The model under review builds one solid part; all positions refer to its coordinate system, in mm. A direction names the side the tool comes from. Give positions to 0.01 mm unless a question says otherwise; leave off trailing zeros. Loops run counter-clockwise (first coordinate to the right, second up) from the corner with the lowest first, then second, coordinate; pieces in that order, holes last. Notation, with made-up numbers: (-1.5, 10) - (12.5, 10) arc R8 ccw to (12.5, 21) - close; hole circle Ø8 at (-2.5, -20.75). An arc over 180 degrees is marked (long way). Return JSON: item names as keys, results as strings. Group by question number.
Autodesk Inventor part; units mm, degrees
ref_plane "YZ Plane" through (0, 0, 0) normal (1, 0, 0) x (0, 1, 0)
ref_plane "XZ Plane" through (0, 0, 0) normal (0, 1, 0) x (-1, 0, 0)
ref_plane "XY Plane" through (0, 0, 0) normal (0, 0, 1) x (1, 0, 0)
sketch "Sketch1" plane through (0, 0, 0) normal (0, 1, 0) x (-1, 0, 0)
  line L0 (0, 0) -> (25, 0)
  line L1 (25, 0) -> (25, -30)
  line L2 (25, -30) -> (0, -30)
  line L3 (0, -30) -> (0, 0)
  circle A0 centre (20, -4) radius 1.5
  circle A1 centre (20, -26) radius 1.5
  circle A2 centre (10, -4) radius 1.5
  circle A3 centre (10, -26) radius 1.5
  dimension "d0" = 30
  dimension "d1" = 25
  dimension "d2" = 3
  dimension "d5" = 22
  dimension "d8" = 10
  dimension "d11" = 20
  dimension "d12" = 4
extrude "Extrusion1" add sketch "Sketch1" along normal blind 25.5
sketch "Sketch2" plane through (0, 0, 0) normal (1, 0, 0) x (0, 0, -1)
  line L0 (0, 0) -> (30, 0)
  line L1 (30, 0) -> (30, 25.5)
  line L2 (0, 25.5) -> (30, 25.5)
  line L3 (0, 0) -> (0, 25.5)
  line L4 (8.25, 25.5) -> (21.75, 25.5)
  line L5 (21.75, 25.5) -> (21.75, 3)
  line L6 (21.75, 3) -> (8.25, 3)
  line L7 (8.25, 3) -> (8.25, 25.5)
  line L8 (30, 25.5) -> (0, 25.5)
  line L9 (30, 0) -> (30, 25.5)
  line L10 (24.15, 25.5) -> (30, 25.5)
  line L11 (30, 25.5) -> (30, 3)
  line L12 (30, 3) -> (24.15, 3)
  line L13 (24.15, 3) -> (24.15, 25.5)
  line L14 (0, 25.5) -> (5.85, 25.5)
  line L15 (5.85, 25.5) -> (5.85, 3)
  line L16 (5.85, 3) -> (0, 3)
  line L17 (0, 3) -> (0, 25.5)
  point P0 (0, 3)
  point P1 (30, 3)
  dimension "d15" = 3
  dimension "d16" = 3
  dimension "d17" = 3
  dimension "d19" = 13.5
  dimension "d20" = 2.4
  dimension "d21" = 2.4
  dimension "d22" = 5.85
extrude "Extrusion2" cut sketch "Sketch2" against normal blind 25.5 contours L3 L2 L15 L16 | L12 L13 L2 L1 | L2 L5 L6 L7
sketch "Sketch3" plane through (0, 3, -5.85) normal (0, 0, 1) x (1, 0, 0)
  circle A0 centre (-18, 8) radius 5
  line L0 (-25, 0) -> (-25, 22.5)
  line L1 (0, 0) -> (-25, 0)
  line L2 (0, 22.5) -> (0, 0)
  line L3 (-25, 22.5) -> (0, 22.5)
  line L4 (-25, 15) -> (-11, 15)
  line L5 (-11, 15) -> (0, 6)
  line L6 (0, 0) -> (0, 22.5)
  point P0 (0, -3)
  point P1 (0, 6)
  dimension "d25" = 8
  dimension "d26" = 7
  dimension "d27" = 7
  dimension "d28" = 14
  dimension "d29" = 6
  dimension "d30" = 10
extrude "Extrusion3" cut sketch "Sketch3" against normal blind 25.5 contours A0 | L0 L3 L2 L5 L4
fillet "Fillet1" radius 7 6 edges at (-25, 18, -22.95) (-11, 18, -22.95) (0, 9, -22.95) (-11, 18, -7.05) (0, 9, -7.05) (-25, 18, -7.05)
properties part number "beslag_board_3D"
Item 1: For L1, parallel to Z at x = -10, y = 1.25; L2, parallel to X at y = 1.05, z = -4; L3, parallel to Y at x = -18, z = -7.2, list the stretches that pass through material, from the lowest coordinate up. Write a range as from..to.
Item 2: Mouldability with a two-part tool opening along Y and no side actions: class faces 1 (the face through (-12, 9, -8.25)), 2 (the face through (-12, 3, -3)), 3 (the face through (-22, 14, -23)) as +Y half, -Y half, draft (parallel to the pull), parting line (faces both ways), or undercut.
Item 3: Take a section at C-C (z = -22.5). State the section outline as (x, y) points.
Item 4: Take a section at B-B (y = 13.5). State the section outline as (x, z) points.
Item 5: Take a section at A-A (z = -26). State the section outline as (x, y) points, then the cut area to 3 significant figures.
Item 6: Take a section at D-D (y = 1.75). State the section outline as (x, z) points, then the cut area to 3 significant figures.
Item 7: For P1, Ø3, axis at x = -21.5, y = 5.5, coming from the -Z side; P2, Ø3.5, axis at x = -10, z = -4, coming from the +Y side; P3, Ø5, axis at x = -10, z = -26, coming from the +Y side, all flat-tipped, find the tip position at first contact; note any pin that passes through.
Item 8: Tool access review of faces 4 (the face through (-12, 1, 0)), 5 (the face through (-12, 3, -27)), 6 (the face through (-11.177, 17.604, -7.067)), 7 (the face through (-12, 9, -5.85)), 8 (the face through (-12, 9, -21.75)): name each direction out of +Z, -Z, +X, -X, +Y, -Y from which nothing blocks a thin tool from reaching the whole face with its end or side.
Check sheet entries:
{
 "1": {"L1": "z = -30..-27.5, -24.5..-5.5, -2.5..0", "L2": "x = -25..-21.5, -18.5..-11.5, -8.5..0", "L3": "y = 0..6, 16..18"},
 "2": {"face 1": "draft", "face 2": "+Y half", "face 3": "undercut"},
 "3": {"outline": "(-25, 0) - (0, 0) - (0, 5.68) arc R7 ccw to (-2.57, 11.1) - (-9.07, 16.42) arc R7 ccw to (-13.5, 18) - (-18, 18) arc R7 ccw to (-25, 11) - close; hole circle Ø10 at (-18, 11)"},
 "4": {"outline": "(-24.54, -24.15) - (-22.33, -24.15) - (-22.33, -21.75) - (-24.54, -21.75) - close; (-24.54, -8.25) - (-22.33, -8.25) - (-22.33, -5.85) - (-24.54, -5.85) - close; (-13.67, -24.15) - (-5.5, -24.15) - (-5.5, -21.75) - (-13.67, -21.75) - close; (-13.67, -8.25) - (-5.5, -8.25) - (-5.5, -5.85) - (-13.67, -5.85) - close"},
 "5": {"outline": "(-25, 0) - (-21.5, 0) - (-21.5, 3) - (-25, 3) - close; (-18.5, 0) - (-11.5, 0) - (-11.5, 3) - (-18.5, 3) - close; (-8.5, 0) - (0, 0) - (0, 3) - (-8.5, 3) - close", "area": "57.0 mm^2"},
 "6": {"outline": "(-25, -30) - (0, -30) - (0, 0) - (-25, 0) - close; hole circle Ø3 at (-20, -26); hole circle Ø3 at (-20, -4); hole circle Ø3 at (-10, -26); hole circle Ø3 at (-10, -4)", "area": "722 mm^2"},
 "7": {"P1": "stops at z = -24.15", "P2": "stops at y = 3", "P3": "stops at y = 17.76"},
 "8": {"face 4": "+Z, +X, -X, +Y, -Y", "face 5": "-Z, +X, -X, +Y", "face 6": "+Z, -Z, +X, +Y", "face 7": "+Z, +X, -X, +Y", "face 8": "+X, -X, +Y"}
}
